Geometry check sheet. Reference: the model listing, model coordinates, mm. Round coordinates to 2 decimals unless told otherwise and drop trailing zeros. Order: outer loops, then holes, each group sorted by start corner. A loop starts at its lowest first (then second) coordinate and runs counter-clockwise, first axis right, second up. Notation, with made-up numbers: M 88.25,87.25 L 95.25,87.25 A24 ccw 95.25,98.25 Z; hole C 22.25,14 d4. An arc over 180 degrees is marked long. Return JSON: item names as keys, results as strings. Group by question number.
```python
from build123d import *

# Parameters (mm, degrees)
SKETCH1_R          = 381
SKETCH1_R_2        = 342.9
EXTRUDE1_DEPTH     = 2.032
SKETCH2_R          = 3.556
CUT_EXTRUDE1_DEPTH = 2.032
CIRPATTERN1_COUNT  = 10


with BuildPart() as part:
    # Sketch1 → Extrude1 (new body)
    with BuildSketch(Plane.XY):
        Circle(SKETCH1_R)
        Circle(SKETCH1_R_2, mode=Mode.SUBTRACT)
    extrude(amount=EXTRUDE1_DEPTH)

    # Sketch2 → Cut-Extrude1 (cut)
    with BuildSketch(Plane.XY.offset(2.032)):
        with Locations((0, -361.95)):
            Circle(SKETCH2_R)
    cut_extrude1 = extrude(amount=-CUT_EXTRUDE1_DEPTH, mode=Mode.SUBTRACT)

    # CirPattern1: Cut-Extrude1 ×10 about axis
    cirpattern1_axis = Axis((0, 0, 0), (0, 0, 1))
    for i in range(1, CIRPATTERN1_COUNT):
        add(cut_extrude1.rotate(cirpattern1_axis, i * 360 / CIRPATTERN1_COUNT), mode=Mode.SUBTRACT)


solid = part.part
```
Q1. Depth check by flat-ended pin: pin 1 Ø9 at (x, y) = (212.75, 292.82) entering from -Z; pin 2 Ø1 at (y, z) = (13, 1.5) entering from -X. Enter the tip coordinate at first touch or a pass-through.
Q2. Release check for a two-part mould opening along X. For faces 1 (the face through (184.341, 289.135, 1.002)), 2 (the face through (-302.35, -231.83, 1)), 3 (the face through (-312, 143, 0)) record: +X half, -X half, draft (parallel to the pull), parting line (faces both ways), or undercut.
Q3. Section check C-C on z = 1.4. Count the separate pieces of the cut face and the enclosed holes in it, plus the area to 3 significant figures.
Q4. Section check A-A on y = 0. Record the cut outline in (x, z).
Q5. Section check B-B on x = -38.5. Record the cut outline in (y, z), plus the area to 3 significant figures.
Q6. Material ranges on line 1 along Y through (x, z) = (0, 1.1); line 2 along X through (y, z) = (115, 0.15); line 3 along Y through (x, z) = (-124.5, 0.2), recorded low to high.
Geometry check:
{
 "1": {"pin 1": "stops at z = 0", "pin 2": "stops at x = -380.79"},
 "2": {"face 1": "undercut", "face 2": "parting line", "face 3": "draft"},
 "3": {"separate pieces": "1", "enclosed holes": "11", "area": "86,200 mm^2"},
 "4": {"outline": "M -381,0 L -342.9,0 L -342.9,2.03 L -381,2.03 Z; M 342.9,0 L 381,0 L 381,2.03 L 342.9,2.03 Z"},
 "5": {"outline": "M -379.05,0 L -340.73,0 L -340.73,2.03 L -379.05,2.03 Z; M 340.73,0 L 379.05,0 L 379.05,2.03 L 340.73,2.03 Z", "area": "156 mm^2"},
 "6": {"line 1": "y = -381 to -365.51, -358.39 to -342.9, 342.9 to 358.39, 365.51 to 381", "line 2": "x = -363.23 to -345.88, -342.59 to -323.04, 323.04 to 342.59, 345.88 to 363.23", "line 3": "y = -360.08 to -319.5, 319.5 to 360.08"}
}
